Geometry: final body of the model. Coordinates: model frame, mm. Give positions to 0.01 mm unless a question says otherwise; leave off trailing zeros. Write each loop counter-clockwise with the first axis right and the second up, starting at its lowest first coordinate (ties: lowest second). Pieces come first, ordered by that corner, then holes.
from build123d import *

# Parameters (mm, degrees)
SKETCH1_R           = 1.524
BOSS_EXTRUDE1_DEPTH = 6.35
FILLET1_R           = 0.254


with BuildPart() as part:
    # Sketch1 → Boss-Extrude1 (new body)
    with BuildSketch(Plane(origin=(0, 0, 0), x_dir=(1, 0, 0), z_dir=(0, 1, 0))):
        with BuildLine():
            Line((-0.774889862, 9.493427764), (-117.081961553, 0))
            Line((-117.081961553, 0), (-0.774889862, -9.493427764))
            ThreePointArc((-0.774889862, -9.493427764), (2.47998519, -9.19648294), (5.442857143, -7.816708458))
            ThreePointArc((5.442857143, -7.816708458), (12.7, -5.538986403), (19.957142857, -7.816708458))
            ThreePointArc((19.957142857, -7.816708458), (34.925, 0), (19.957142857, 7.816708458))
            ThreePointArc((19.957142857, 7.816708458), (12.7, 5.538986403), (5.442857143, 7.816708458))
            ThreePointArc((5.442857143, 7.816708458), (2.47998519, 9.19648294), (-0.774889862, 9.493427764))
        make_face()
        Circle(SKETCH1_R, mode=Mode.SUBTRACT)
        with Locations((25.4, 0)):
            Circle(SKETCH1_R, mode=Mode.SUBTRACT)
    extrude(amount=BOSS_EXTRUDE1_DEPTH)

    # Fillet1
    fillet1_edges = [part.edges().sort_by_distance(p)[0] for p in [
        (-117.081961553, 3.175, 0),
    ]]
    fillet(fillet1_edges, radius=FILLET1_R)


solid = part.part
Q1. Pull-direction query (X, two-part tool) for faces 1 (the flat face through (-24, 6.35, 0)), 2 (the cylindrical face through (12.81, 3.13, -5.54)), 3 (the flat face through (-56.585, 3.131, -4.938)); classes: released by +X, released by -X, zero draft, split by the parting line, or undercut.
Filled sheet:
face 1: zero draft
face 2: undercut
face 3: released by -X
Q2. Section C-C on x = 7.5. Output: boundary loops of the cut face in (y, z).
Filled sheet:
outline: (0, -6.65) - (6.35, -6.65) - (6.35, 6.65) - (0, 6.65) - close
Q3. Section A-A on x = 25.4. Output: boundary loops of the cut face in (y, z) (3 decimals), plus the area to 3 significant figures.
Filled sheet:
outline: (0, -9.525) - (6.35, -9.525) - (6.35, -1.524) - (0, -1.524) - close; (0, 1.524) - (6.35, 1.524) - (6.35, 9.525) - (0, 9.525) - close
area: 102 mm2
Q4. Pin query (flat end, axial travel): P1, Ø3, axis at y = 4, z = -3, coming from the +X side; P2, Ø2.5, axis at x = 0, z = 0, coming from the +Y side. Return the tip coordinate at first contact, or that it passes through.
Filled sheet:
P1: stops at x = 34.81
P2: passes through
Q5. Section D-D on x = -40. Output: boundary loops of the cut face in (y, z), plus the area to 3 significant figures.
Filled sheet:
outline: (0, -6.29) - (6.35, -6.29) - (6.35, 6.29) - (0, 6.29) - close
area: 79.9 mm2
Q6. Section B-B on y = 2.5. Output: boundary loops of the cut face in (x, z) (3 decimals), plus the area to 3 significant figures.
Filled sheet:
outline: (-113.98, -0.253) - (-0.775, -9.493) arc R9.525 ccw to (5.443, -7.817) arc R12.7 cw to (19.957, -7.817) arc R9.525 ccw (long way) to (19.957, 7.817) arc R12.7 cw to (5.443, 7.817) arc R9.525 ccw to (-0.775, 9.493) - (-113.98, 0.253) arc R0.254 ccw to start; hole circle Ø3.048 at (0, 0); hole circle Ø3.048 at (25.4, 0)
area: 1,620 mm2
Q7. Ray query, line 1 along Z through (x, y) = (25.4, 5.25) (3 decimals); line 2 along Z through (x, y) = (-21, 1); line 3 along Z through (x, y) = (-31, 3.75). Return the intervals inside material, ascending.
Filled sheet:
line 1: z = -9.525 to -1.524, 1.524 to 9.525
line 2: z = -7.84 to 7.84
line 3: z = -7.03 to 7.03
